Read the model definition and answer for the solid it produces. Units are mm, in the model's axes. A direction names the side the tool comes from. Coordinates: 2 decimals unless noted, no trailing zeros. Loops run counter-clockwise (first coordinate to the right, second up) from the corner with the lowest first, then second, coordinate; pieces in that order, holes last.
Q1. Section C-C (z = 76.5) is taken. Give the vertices of the cut face in (x, y), then the cut area to 3 significant figures.
Q2. Section B-B (x = 14) is taken. Give the vertices of the cut face in (y, z).
Q3. Straight lines are drawn through the part: line 1 (Y direction, x = 0, z = 52); line 2 (Y direction, x = -25.5, z = 39). For each, find the intervals that lie inside material, in ascending order.
Q4. Which of the six approach directions +Z, -Z, +X, -X, +Y, -Y give full straight-line access (tool end or side, diameter ignored) to faces 1 (the face through (0, 51, 3)), 2 (the face through (54.89, 17.29, 1.52))?
Q5. Flat-ended cylindrical pins translate along their axes: P1, Ø5, axis at x = -41, z = 57.5, coming from the +Y side; P2, Ø12, axis at y = 4, z = 22, coming from the +X side; P3, Ø4, axis at y = -14, z = 29, coming from the +X side (3 decimals); P4, Ø5, axis at x = -23.5, y = 45.5, coming from the -Z side. Find the tip coordinate at first contact, or state that the pin passes through.
Q6. The mould has two halves that part along X. Classify faces 3 (the face through (-22, -43, 0)), 4 (the face through (-10.958, -49.348, 43.56)): pulls with the +X half, pulls with the -X half, needs draft (parallel to the pull), parting line crosses it, or undercut.
Q7. Section A-A (y = -26) is taken. Give the vertices of the cut face in (x, z), then the cut area to 3 significant figures.
from build123d import *

# Parameters (mm, degrees)
REVOLUTION_ANGLE            = 90
REVOLUTION_MIRRORED_2_ANGLE = -90


with BuildPart() as part:
    # Sketch → Revolution (revolve)
    with BuildSketch(Plane.XZ):
        Polygon((47.55, 0), (50.55, 0), (57.55, 0), (57.55, 3), (50.55, 3), (50.55, 83), (47.55, 83), align=None)
    revolution = revolve(axis=Axis((0, 0, 0), (0, 0, 1)), revolution_arc=REVOLUTION_ANGLE)

    # Sketch Mirrored 2 → Revolution Mirrored 2 (revolve)
    with BuildSketch(Plane(origin=(0, 0, 0), x_dir=(-1, 0, 0), z_dir=(0, 1, 0))):
        Polygon((47.55, 0), (50.55, 0), (57.55, 0), (57.55, 3), (50.55, 3), (50.55, 83), (47.55, 83), align=None)
    revolution_mirrored_2 = revolve(axis=Axis((0, 0, 0), (0, 0, 1)), revolution_arc=REVOLUTION_MIRRORED_2_ANGLE)

    # Mirrored001: Revolution, Revolution Mirrored 2 across Sketch001 H_Axis
    add(revolution.mirror(Plane.ZX))
    add(revolution_mirrored_2.mirror(Plane.ZX))


solid = part.part
Numbers:
1. outline: circle Ø101.1 at (0, 0); hole circle Ø95.1 at (0, 0)
1. area: 925 mm2
2. outline: (-55.82, 0) - (-45.44, 0) - (-45.44, 83) - (-48.57, 83) - (-48.57, 3) - (-55.82, 3) - close; (45.44, 0) - (55.82, 0) - (55.82, 3) - (48.57, 3) - (48.57, 83) - (45.44, 83) - close
3. line 1: y = -50.55 to -47.55, 47.55 to 50.55
3. line 2: y = -43.65 to -40.13, 40.13 to 43.65
4. face 1: +Z
4. face 2: +Z, -Z
5. P1: stops at y = 32.76
5. P2: stops at x = 50.55
5. P3: stops at x = 49.105
5. P4: stops at z = 0
6. face 3: needs draft
6. face 4: parting line crosses it
7. outline: (-51.34, 0) - (-39.81, 0) - (-39.81, 83) - (-43.35, 83) - (-43.35, 3) - (-51.34, 3) - close; (39.81, 0) - (51.34, 0) - (51.34, 3) - (43.35, 3) - (43.35, 83) - (39.81, 83) - close
7. area: 635 mm2
